```python
from build123d import *

# Parameters (mm, degrees)
BOSS_EXTRUDE2_DEPTH  = 8
SKETCH3_R            = 5.25
CUT_EXTRUDE1_DEPTH   = 8
SKETCH7_W            = 4
SKETCH7_H            = 9
BOSS_EXTRUDE3_DEPTH  = 8
SKETCH8_W            = 4
SKETCH8_H            = 40
BOSS_EXTRUDE4_DEPTH  = 12
SKETCH9_W            = 20
SKETCH9_H            = 4
BOSS_EXTRUDE5_DEPTH  = 24
SKETCH10_W           = 20
SKETCH10_H           = 4
BOSS_EXTRUDE6_DEPTH  = 24
SKETCH12_W           = 4
SKETCH12_H           = 38
BOSS_EXTRUDE7_DEPTH  = 20
SKETCH13_W           = 4
SKETCH13_H           = 20
BOSS_EXTRUDE8_DEPTH  = 12
SKETCH14_R           = 1.5
CUT_EXTRUDE2_DEPTH   = 12
SKETCH15_R           = 1.5
CUT_EXTRUDE3_DEPTH   = 12
FILLET1_R            = 3
SKETCH16_R           = 1.5
CUT_EXTRUDE4_DEPTH   = 12
SKETCH21_W           = 8
SKETCH21_H           = 22
BOSS_EXTRUDE9_DEPTH  = 20
SKETCH22_R           = 11
BOSS_EXTRUDE10_DEPTH = 8
SKETCH23_R           = 1.5
SKETCH23_R_2         = 5.25
CUT_EXTRUDE6_DEPTH   = 21
SKETCH24_R           = 1.5
SKETCH24_R_2         = 5.25
CUT_EXTRUDE7_DEPTH   = 8


with BuildPart() as part:
    # Sketch1 → Boss-Extrude2 (new body)
    with BuildSketch(Plane.XY):
        with BuildLine():
            ThreePointArc((12, 11), (1, 0), (12, -11))
            Line((12, -11), (12, 11))
        make_face()
        with BuildLine():
            Line((12, 11), (12, -11))
            ThreePointArc((12, -11), (19.778174593, -7.778174593), (23, 0))
            ThreePointArc((23, 0), (19.778174593, 7.778174593), (12, 11))
        make_face()
        with BuildLine():
            Line((-12, 11), (-12, -11))
            Line((-12, -11), (12, -11))
            ThreePointArc((12, -11), (1, 0), (12, 11))
            Line((12, 11), (-12, 11))
        make_face()
    extrude(amount=BOSS_EXTRUDE2_DEPTH)

    # Sketch3 → Cut-Extrude1 (cut)
    with BuildSketch(Plane.XY.offset(8)):
        with Locations((12, 0)):
            Circle(SKETCH3_R)
    extrude(amount=-CUT_EXTRUDE1_DEPTH, mode=Mode.SUBTRACT)

    # Sketch7 → Boss-Extrude3 (add)
    with BuildSketch(Plane.XY.offset(8)):
        with Locations((-10, 15.5)):
            Rectangle(SKETCH7_W, SKETCH7_H)
        with Locations((-10, -15.5)):
            Rectangle(SKETCH7_W, SKETCH7_H)
    extrude(amount=-BOSS_EXTRUDE3_DEPTH)

    # Sketch8 → Boss-Extrude4 (add)
    with BuildSketch(Plane(origin=(0, 0, 0), x_dir=(-1, 0, 0), z_dir=(0, 0, -1))):
        with Locations((10, 0)):
            Rectangle(SKETCH8_W, SKETCH8_H)
    extrude(amount=BOSS_EXTRUDE4_DEPTH)

    # Sketch9 → Boss-Extrude5 (add)
    with BuildSketch(Plane.ZY.offset(12)):
        with Locations((-2, 18)):
            Rectangle(SKETCH9_W, SKETCH9_H)
    extrude(amount=BOSS_EXTRUDE5_DEPTH)

    # Sketch10 → Boss-Extrude6 (add)
    with BuildSketch(Plane.ZY.offset(12)):
        with Locations((-2, -18)):
            Rectangle(SKETCH10_W, SKETCH10_H)
    extrude(amount=BOSS_EXTRUDE6_DEPTH)

    # Sketch12 → Boss-Extrude7 (add)
    with BuildSketch(Plane(origin=(0, 0, -12), x_dir=(-1, 0, 0), z_dir=(0, 0, -1))):
        with Locations((34, 39)):
            Rectangle(SKETCH12_W, SKETCH12_H)
    extrude(amount=-BOSS_EXTRUDE7_DEPTH)

    # Sketch13 → Boss-Extrude8 (add)
    with BuildSketch(Plane.XZ.offset(20)):
        with Locations((-34, -2)):
            Rectangle(SKETCH13_W, SKETCH13_H)
    extrude(amount=BOSS_EXTRUDE8_DEPTH)

    # Sketch14 → Cut-Extrude2 (cut)
    with BuildSketch(Plane.ZY.offset(36)):
        with Locations((-2, -27.5)):
            Circle(SKETCH14_R)
    extrude(amount=-CUT_EXTRUDE2_DEPTH, mode=Mode.SUBTRACT)

    # Sketch15 → Cut-Extrude3 (cut)
    with BuildSketch(Plane.ZY.offset(36)):
        with Locations((-2, 51)):
            Circle(SKETCH15_R)
        with Locations((-2, 44)):
            Circle(SKETCH15_R)
        with Locations((-2, 37)):
            Circle(SKETCH15_R)
        with Locations((-2, 30)):
            Circle(SKETCH15_R)
    extrude(amount=-CUT_EXTRUDE3_DEPTH, mode=Mode.SUBTRACT)

    # Fillet1
    fillet1_edges = [part.edges().sort_by_distance(p)[0] for p in [
        (-34, -32, -12),
        (-34, -32, 8),
        (-34, 58, 8),
        (-34, 58, -12),
    ]]
    fillet(fillet1_edges, radius=FILLET1_R)

    # Sketch16 → Cut-Extrude4 (cut)
    with BuildSketch(Plane(origin=(0, 0, 0), x_dir=(-1, 0, 0), z_dir=(0, 0, -1))):
        with Locations((-12, 8.5)):
            Circle(SKETCH16_R)
        with Locations((-20.5, 0)):
            Circle(SKETCH16_R)
        with Locations((-12, -8.5)):
            Circle(SKETCH16_R)
        with Locations((-3.5, 0)):
            Circle(SKETCH16_R)
    extrude(amount=-CUT_EXTRUDE4_DEPTH, mode=Mode.SUBTRACT)

    # Sketch21 → Boss-Extrude9 (add)
    with BuildSketch(Plane(origin=(-8, 0, 0), x_dir=(0, 0, -1), z_dir=(1, 0, 0))):
        with Locations((8, 0)):
            Rectangle(SKETCH21_W, SKETCH21_H)
    extrude(amount=BOSS_EXTRUDE9_DEPTH)

    # Sketch22 → Boss-Extrude10 (add)
    with BuildSketch(Plane(origin=(0, 0, -12), x_dir=(-1, 0, 0), z_dir=(0, 0, -1))):
        with Locations((-12, 0)):
            Circle(SKETCH22_R)
    extrude(amount=-BOSS_EXTRUDE10_DEPTH)

    # Sketch23 → Cut-Extrude6 (cut, through all)
    with BuildSketch(Plane.XY.offset(8)):
        with Locations((12, 8.5)):
            Circle(SKETCH23_R)
        with Locations((20.5, 0)):
            Circle(SKETCH23_R)
        with Locations((3.5, 0)):
            Circle(SKETCH23_R)
        with Locations((12, -8.5)):
            Circle(SKETCH23_R)
        with Locations((12, 0)):
            Circle(SKETCH23_R_2)
    extrude(amount=-CUT_EXTRUDE6_DEPTH, mode=Mode.SUBTRACT)

    # Sketch24 → Cut-Extrude7 (cut)
    with BuildSketch(Plane.XY.offset(8)):
        with BuildLine():
            Line((12, 11), (-8, 11))
            Line((-8, 11), (-8, -11))
            Line((-8, -11), (12, -11))
            ThreePointArc((12, -11), (1, 0), (12, 11))
        make_face()
        with BuildLine():
            Line((12, 10), (12, 11))
            ThreePointArc((12, 11), (1, 0), (12, -11))
            Line((12, -11), (12, -10))
            ThreePointArc((12, -10), (10.5, -8.5), (12, -7))
            Line((12, -7), (12, -5.25))
            ThreePointArc((12, -5.25), (6.75, 0), (12, 5.25))
            Line((12, 5.25), (12, 7))
            ThreePointArc((12, 7), (10.5, 8.5), (12, 10))
        make_face()
        with Locations((3.5, 0)):
            Circle(SKETCH24_R, mode=Mode.SUBTRACT)
        with Locations((12, 8.5)):
            Circle(SKETCH24_R)
        with Locations((12, 0)):
            Circle(SKETCH24_R_2)
        with Locations((12, -8.5)):
            Circle(SKETCH24_R)
        with BuildLine():
            Line((12, 11), (12, -11))
            ThreePointArc((12, -11), (23, 0), (12, 11))
        make_face()
        with Locations((20.5, 0)):
            Circle(SKETCH24_R, mode=Mode.SUBTRACT)
    extrude(amount=-CUT_EXTRUDE7_DEPTH, mode=Mode.SUBTRACT)


solid = part.part
```
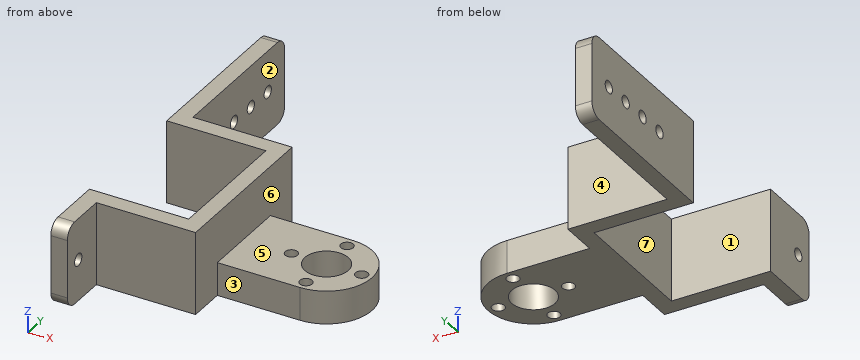
The model under review builds one solid part; all positions refer to its coordinate system, in mm. Face numbers are marked on the shaded views. A direction names the side the tool comes from. Round coordinates to 2 decimals unless told otherwise and drop trailing zeros. Loops run counter-clockwise (first coordinate to the right, second up) from the corner with the lowest first, then second, coordinate; pieces in that order, holes last. Notation, with made-up numbers: (49, 68) -> (104, 68) arc R30 cw to (104, 99) -> close; hole circle Ø5 at (-4, 12.25). An arc over 180 degrees is marked (long way). Answer as a JSON object with one key per item and string values. Group by question number.
1) We need section B-B on y = 0. Write out the cut boundary in (x, z), then the cut area to 3 significant figures.
2) For pin 1 Ø24 at (x, y) = (10.5, -1) entering from +Z; pin 2 Ø10 at (x, z) = (-8.5, -6.5) entering from -Y; pin 3 Ø1.5 at (x, z) = (-12.5, 1.5) entering from +Y, all flat-tipped, find the tip position at first contact; note any pin that passes through.
3) We need section C-C on z = -5.5. Write out the cut boundary in (x, y), then the cut area to 3 significant figures.
4) Mouldability with a two-part tool opening along Y and no side actions: class the marked faces 1, 2 and 3 as released by +Y, released by -Y, zero draft, split by the parting line, or undercut.
5) We need section D-D on y = 44. Write out the cut boundary in (x, z).
6) For the marked faces 4, 5, 6 and 7, list the 3-axis set-ups (+Z, -Z, +X, -X, +Y, -Y) from which the entire face can be reached by the end or side of a thin tool; tool diameter is ignored.
7) For line 1 (Y direction, x = -33, z = -7.25); line 2 (Y direction, x = 3.5, z = -8.25); line 3 (X direction, y = 32, z = -6.5), list the stretches that pass through material, from the lowest coordinate up. Write a range as [from, to].
8) We need section A-A on x = -15. Write out the cut boundary in (y, z).
Result set:
{
 "1": {"outline": "(-12, -12) -> (2, -12) -> (2, -4) -> (-8, -4) -> (-8, 8) -> (-12, 8) -> close; (5, -12) -> (6.75, -12) -> (6.75, -4) -> (5, -4) -> close; (17.25, -12) -> (19, -12) -> (19, -4) -> (17.25, -4) -> close; (22, -12) -> (23, -12) -> (23, -4) -> (22, -4) -> close", "area": "196 mm²"},
 "2": {"pin 1": "z = -4", "pin 2": "y = -20", "pin 3": "y = 20"},
 "3": {"outline": "(-36, -32) -> (-32, -32) -> (-32, -20) -> (-8, -20) -> (-8, -11) -> (12, -11) arc R11 ccw to (12, 11) -> (-8, 11) -> (-8, 20) -> (-32, 20) -> (-32, 58) -> (-36, 58) -> (-36, 16) -> (-12, 16) -> (-12, -16) -> (-36, -16) -> close; hole circle Ø3 at (3.5, 0); hole circle Ø10.5 at (12, 0); hole circle Ø3 at (12, -8.5); hole circle Ø3 at (12, 8.5); hole circle Ø3 at (20.5, 0)", "area": "1,070 mm²"},
 "4": {"face 1": "undercut", "face 2": "zero draft", "face 3": "released by -Y"},
 "5": {"outline": "(-36, -12) -> (-32, -12) -> (-32, -3.5) -> (-36, -3.5) -> close; (-36, -0.5) -> (-32, -0.5) -> (-32, 8) -> (-36, 8) -> close"},
 "6": {"face 4": "+Z, -Z, +X, +Y", "face 5": "+Z, +X, +Y, -Y", "face 6": "+Z, +X", "face 7": "+Z, -Z, -X"},
 "7": {"line 1": "[-32, -16], [16, 58]", "line 2": "[-11, -1.5], [1.5, 11]", "line 3": "[-36, -32]"},
 "8": {"outline": "(-20, -12) -> (-16, -12) -> (-16, 8) -> (-20, 8) -> close; (16, -12) -> (20, -12) -> (20, 8) -> (16, 8) -> close"}
}
